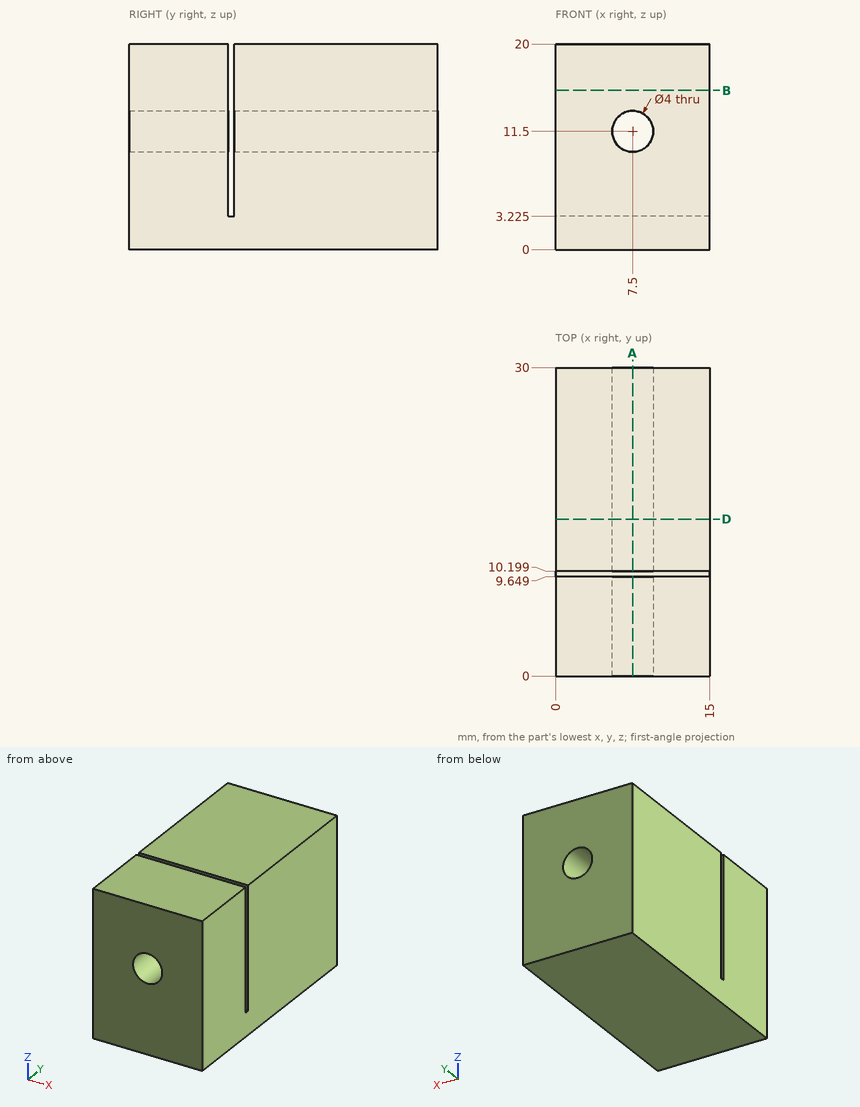
Can you work these out from the drawing? Everything is in mm from the part's minimum corner. Coordinates: 2 decimals unless noted, no trailing zeros. Loops run counter-clockwise (first coordinate to the right, second up) from the corner with the lowest first, then second, coordinate; pieces in that order, holes last. Notation, with made-up numbers: (-9, 84) - (-2, 84) arc R6 cw to (-2, 92) - close; hole circle Ø7 at (40, 32.5). An arc over 180 degrees is marked (long way). Use a Markdown table: item, result.
Item 1: I want a section at B-B on z = 15.5. Please give me the cut outline in (x, y), and give its area (3 significant figures).
Numbers:
| item | result |
|---|---|
| outline | (0, 0) - (15, 0) - (15, 9.65) - (0, 9.65) - close; (0, 10.2) - (15, 10.2) - (15, 30) - (0, 30) - close |
| area | 442 mm2 |
Item 2: I want a section at D-D on y = 15.25. Please give me the cut outline in (x, z).
Numbers:
| item | result |
|---|---|
| outline | (0, 0) - (15, 0) - (15, 20) - (0, 20) - close; hole circle Ø4 at (7.5, 11.5) |
Item 3: If I drill on probe 1 along Y at (x, z) = (13.5, 9.75); probe 2 along Z at (x, y) = (7.5, 24.25); probe 3 along Z at (x, y) = (8.75, 21), over which ranges is the centre line in solid material (lowest first)? Write a range as from..to.
Numbers:
| item | result |
|---|---|
| probe 1 | y = 0..9.65, 10.2..30 |
| probe 2 | z = 0..9.5, 13.5..20 |
| probe 3 | z = 0..9.94, 13.06..20 |
Item 4: I want a section at A-A on x = 7.5. Give the number of separate pieces and of enclosed holes in the cut face, and give its area (3 significant figures).
Numbers:
| item | result |
|---|---|
| separate pieces | 3 |
| enclosed holes | 0 |
| area | 473 mm2 |
